Geometry check sheet. Reference: the model listing, model coordinates, mm. Face numbers are marked on the shaded views. A direction names the side the tool comes from. Coordinates: 2 decimals unless noted, no trailing zeros. Write each loop counter-clockwise with the first axis right and the second up, starting at its lowest first coordinate (ties: lowest second). Pieces come first, ordered by that corner, then holes. Notation, with made-up numbers: (44, 18.5) -> (79, 18.5) arc R21 cw to (79, 32.5) -> close; hole circle Ø2 at (78.5, -22.5). An arc over 180 degrees is marked (long way). Answer in a Markdown table with one row per item. Add a question column.
1. Cross-section at B-B on y = 3. Record the cut outline in (x, z), and give its area (3 significant figures).
2. Cross-section at A-A on x = -13.75. Record the cut outline in (y, z).
3. Cross-section at D-D on z = -4.5. Record the cut outline in (x, y).
4. Set-up check for the marked faces 1, 2 and 3: record each of +Z, -Z, +X, -X, +Y, -Y from which the full face is reachable in a straight line by a thin tool's end or side.
5. Cross-section at C-C on x = -1.5. Record the cut outline in (y, z), and give its area (3 significant figures).
6. Depth check by flat-ended pin: P1, Ø1, axis at x = -7, y = 26.5, coming from the -Z side; P2, Ø2, axis at x = -10, z = -2.5, coming from the +Y side; P3, Ø1, axis at x = 8, z = -1.5, coming from the +Y side. Enter the tip coordinate at first touch or a pass-through.
7. Scan lines: L1, parallel to Z at x = -13.75, y = 17.45; L2, parallel to X at y = 12.5, z = -4.5; L3, parallel to X at y = 17.45, z = 0. Record each from-to range of solid material in increasing order. Write a range as from..to.
```python
from build123d import *

# Parameters (mm, degrees)
SKETCH1_W           = 22.5
SKETCH1_H           = 22.2
BOSS_EXTRUDE1_DEPTH = 6
BOSS_EXTRUDE2_DEPTH = 4
SKETCH3_R           = 2.5
BOSS_EXTRUDE3_DEPTH = 3.5
SKETCH4_W           = 12
SKETCH4_H           = 2.5
BOSS_EXTRUDE4_DEPTH = 16
CUT_EXTRUDE1_DEPTH  = 2.5


with BuildPart() as part:
    # Sketch1 → Boss-Extrude1 (new, symmetric)
    with BuildSketch(Plane.XY):
        with Locations((0, 11.1)):
            Rectangle(SKETCH1_W, SKETCH1_H)
    extrude(amount=BOSS_EXTRUDE1_DEPTH, both=True)

    # Sketch2 → Boss-Extrude2 (add)
    with BuildSketch(Plane(origin=(0, 22.2, 0), x_dir=(1, 0, 0), z_dir=(0, 1, 0))):
        with BuildLine():
            Line((0.946152423, 3), (-0.053847577, 3))
            ThreePointArc((-0.053847577, 3), (-11.25, 0), (-0.053847577, -3))
            Line((-0.053847577, -3), (0.946152423, -3))
            ThreePointArc((0.946152423, -3), (3.946152423, 0), (0.946152423, 3))
        make_face()
    extrude(amount=BOSS_EXTRUDE2_DEPTH)

    # Sketch3 → Boss-Extrude3 (add)
    with BuildSketch(Plane(origin=(0, 26.2, 0), x_dir=(1, 0, 0), z_dir=(0, 1, 0))):
        with Locations(Location((-5.379476527, 0.226239141, 0), (0, 0, 270))):
            Circle(SKETCH3_R)
    extrude(amount=BOSS_EXTRUDE3_DEPTH)

    # Sketch4 → Boss-Extrude4 (add, symmetric)
    with BuildSketch(Plane(origin=(0, 0, 0), x_dir=(0, 0, -1), z_dir=(1, 0, 0))):
        with Locations((0, 17.45)):
            Rectangle(SKETCH4_W, SKETCH4_H)
    extrude(amount=BOSS_EXTRUDE4_DEPTH, both=True)

    # Sketch5 → Cut-Extrude1 (cut)
    with BuildSketch(Plane(origin=(0, 18.7, 0), x_dir=(1, 0, 0), z_dir=(0, 1, 0))):
        with BuildLine():
            Line((14.616025404, 0.5), (16, 0.5))
            Line((16, 0.5), (16, -0.5))
            Line((16, -0.5), (14.616025404, -0.5))
            ThreePointArc((14.616025404, -0.5), (12.75, 0), (14.616025404, 0.5))
        make_face()
    cut_extrude1 = extrude(amount=-CUT_EXTRUDE1_DEPTH, mode=Mode.SUBTRACT)

    # Mirror1: Cut-Extrude1 across plane
    add(cut_extrude1.mirror(Plane(origin=(0, 0, 0), x_dir=(0, 0, 1), z_dir=(1, 0, 0))), mode=Mode.SUBTRACT)


solid = part.part
```
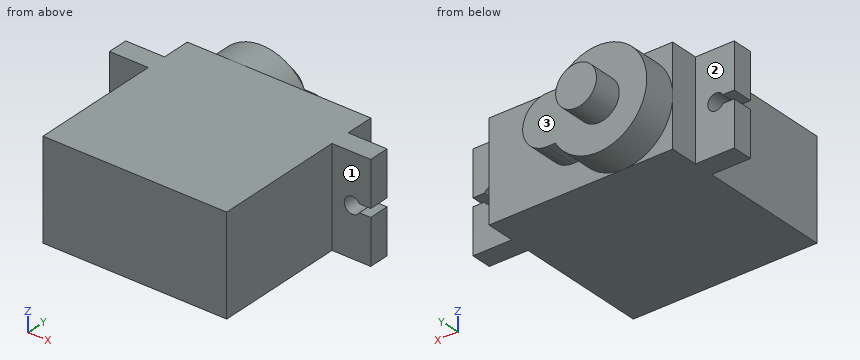
Results found:
| question | item | result |
|---|---|---|
| 1 | outline | (-11.25, -6) -> (11.25, -6) -> (11.25, 6) -> (-11.25, 6) -> close |
| 1 | area | 270 mm^2 |
| 2 | outline | (16.2, -6) -> (18.7, -6) -> (18.7, -1) -> (16.2, -1) -> close; (16.2, 1) -> (18.7, 1) -> (18.7, 6) -> (16.2, 6) -> close |
| 3 | outline | (-16, 16.2) -> (-11.25, 16.2) -> (-11.25, 0) -> (11.25, 0) -> (11.25, 16.2) -> (16, 16.2) -> (16, 18.7) -> (11.25, 18.7) -> (11.25, 22.2) -> (-1.28, 22.2) -> (-1.28, 26.2) -> (-9.22, 26.2) -> (-9.22, 22.2) -> (-11.25, 22.2) -> (-11.25, 18.7) -> (-16, 18.7) -> close |
| 4 | face 1 | +Z, -Z, +X, -Y |
| 4 | face 2 | +Z, -Z, -X, +Y |
| 4 | face 3 | +Y |
| 5 | outline | (0, -6) -> (22.2, -6) -> (22.2, -4.68) -> (26.2, -4.68) -> (26.2, 4.68) -> (22.2, 4.68) -> (22.2, 6) -> (0, 6) -> close |
| 5 | area | 304 mm^2 |
| 6 | P1 | stops at z = -5.85 |
| 6 | P2 | stops at y = 26.2 |
| 6 | P3 | stops at y = 22.2 |
| 7 | L1 | z = -6..-1, 1..6 |
| 7 | L2 | x = -11.25..11.25 |
| 7 | L3 | x = -12.75..12.75 |
